from build123d import *

# Parameters (mm, degrees)
F0_W      = 116.84
F0_H      = 116.840008
F1_DEPTH  = 2.54
F3_DEPTH  = 25.4
F5_DEPTH  = 25.4
F6_R      = 1.976826
F7_DEPTH  = 141.732
F9_DEPTH  = 149.86
F11_DEPTH = 25.4
F10_W     = 23.206993
F10_H     = 32.671138
F12_DEPTH = 25.4


with BuildPart() as f1:
    # F0 (on Top) → F1 (new body)
    with BuildSketch(Plane.XY):
        Rectangle(F0_W, F0_H)
    extrude(amount=F1_DEPTH)

    # F2 (on face) → F3 (join)
    with BuildSketch(Plane.XY.offset(2.54)):
        Polygon((-55.8916, -58.420004), (-55.8916, 0), (-55.8916, 58.420004), (-58.42, 58.420004), (-58.42, -58.420004), align=None)
        Polygon((58.42, 58.420004), (55.886142, 58.420004), (55.886142, 0), (55.886142, -58.420004), (58.42, -58.420004), align=None)
    extrude(amount=F3_DEPTH)

    # F4 (on face) → F5 (cut)
    with BuildSketch(Plane.XY.offset(2.54)):
        Polygon((14.150873, 8.89), (14.150873, 0), (14.150873, -8.89), (25.580873, -8.89), (25.580873, 8.89), align=None)
    extrude(amount=-F5_DEPTH, mode=Mode.SUBTRACT)

    # F6 (on face) → F7 (cut)
    with BuildSketch(Plane.YZ.offset(58.42)):
        with Locations((0, 21.034185)):
            Circle(F6_R)
    extrude(amount=-F7_DEPTH, mode=Mode.SUBTRACT)

    # F8 (on face) → F9 (cut)
    with BuildSketch(Plane.YZ.offset(58.42)):
        Polygon((-58.420004, 2.648506), (-12.702574, 27.94), (-58.420004, 27.94), align=None)
        Polygon((58.420004, 27.94), (12.699459, 27.94), (58.420004, 2.637995), align=None)
    extrude(amount=-F9_DEPTH, mode=Mode.SUBTRACT)

    # F10 (on face) → F11 (cut)
    with BuildSketch(Plane.XY.offset(2.54)):
        Polygon((-44.958197, -8.89), (14.150873, -8.89), (14.150873, 8.89), (-9.05612, 8.89), (-21.754064, 8.89), (-44.958197, 8.89), align=None)
        Polygon((-21.754064, 8.89), (-9.05612, 8.89), (-9.05612, 41.561138), (-15.403662, 41.561138), (-21.754064, 41.561138), align=None)
    extrude(amount=-F11_DEPTH, mode=Mode.SUBTRACT)

    # F10 (on face) → F12 (cut)
    with BuildSketch(Plane.XY.offset(2.54)):
        with Locations((2.547376, 25.225569)):
            Rectangle(F10_W, F10_H)
    extrude(amount=-F12_DEPTH, mode=Mode.SUBTRACT)


solid = f1.part
Work out the finished part from the listing and answer in its coordinate system (mm). A direction names the side the tool comes from. Coordinates: 2 decimals unless noted, no trailing zeros. Loops run counter-clockwise (first coordinate to the right, second up) from the corner with the lowest first, then second, coordinate; pieces in that order, holes last. Notation, with made-up numbers: M 59,-21.75 L 81,-21.75 A12 cw 81,-15.75 Z; hole C 63,-34 d8. An arc over 180 degrees is marked long. Answer in a Markdown table with one row per item. Add a question column.
1. A tool of negligible diameter and unlimited length cuts with its end or side. For faces 4 (the cylindrical face through (-57.1, -0.4, 19.1)), 5 (the flat face through (25.581, 0, 1)), 6 (the flat face through (-55.892, -1, 12)), from which of +Z, -Z, +X, -X, +Y, -Y can it reach the whole face along a straight path? Write none if from no direction.
2. Find section A-A, the plane x = 12.5. Write down the section's boundary in (y, z).
3. Find section C-C, the plane z = 14.5. Write down the section's boundary in (x, y), then the cut area to 3 significant figures.
4. A flat-ended cylindrical pin translates along its axis: P1, Ø5, axis at x = 11, y = -29.5, coming from the +Z side. Find the tip coordinate at first contact, or state that the pin passes through.
5. Find section B-B, the plane y = 0. Write down the section's boundary in (x, z).
6. Consider L1, parallel to X at y = -16, z = 23; L2, parallel to X at y = 8.5, z = 2.25; L3, parallel to Z at x = -57.6, y = 0. Determine where each line is inside the solid, lowest interval first.
7. Find section D-D, the plane y = 27.5. Write down the section's boundary in (x, z), then the cut area to 3 significant figures.
8. The mould has two halves that part along X. Classify faces 1 (the flat face through (57.17, -35.88, 15.12)), 2 (the flat face through (-58.42, 1, 11)), 3 (the flat face through (-21.754, 25, 1)): pulls with the +X half, pulls with the -X half, needs draft (parallel to the pull), parting line crosses it, or undercut.
Reported:
| question | item | result |
|---|---|---|
| 1 | face 4 | +X, -X |
| 1 | face 5 | +Z, -Z |
| 1 | face 6 | +Z, +Y, -Y |
| 2 | outline | M -58.42,0 L -8.89,0 L -8.89,2.54 L -58.42,2.54 Z; M 41.56,0 L 58.42,0 L 58.42,2.54 L 41.56,2.54 Z |
| 3 | outline | M -58.42,-37 L -55.89,-37 L -55.89,36.99 L -58.42,36.99 Z; M 55.89,-37 L 58.42,-37 L 58.42,36.99 L 55.89,36.99 Z |
| 3 | area | 375 mm^2 |
| 4 | P1 | stops at z = 2.54 |
| 5 | outline | M -58.42,0 L -44.96,0 L -44.96,2.54 L -55.89,2.54 L -55.89,19.06 L -58.42,19.06 Z; M -58.42,23.01 L -55.89,23.01 L -55.89,27.94 L -58.42,27.94 Z; M 25.58,0 L 58.42,0 L 58.42,19.06 L 55.89,19.06 L 55.89,2.54 L 25.58,2.54 Z; M 55.89,23.01 L 58.42,23.01 L 58.42,27.94 L 55.89,27.94 Z |
| 6 | L1 | x = -58.42 to -55.89, 55.89 to 58.42 |
| 6 | L2 | x = -58.42 to -44.96, 25.58 to 58.42 |
| 6 | L3 | z = 0 to 19.06, 23.01 to 27.94 |
| 7 | outline | M -58.42,0 L -21.75,0 L -21.75,2.54 L -55.89,2.54 L -55.89,19.75 L -58.42,19.75 Z; M 14.15,0 L 58.42,0 L 58.42,19.75 L 55.89,19.75 L 55.89,2.54 L 14.15,2.54 Z |
| 7 | area | 293 mm^2 |
| 8 | face 1 | needs draft |
| 8 | face 2 | pulls with the -X half |
| 8 | face 3 | undercut |
